```python
from build123d import *

# Parameters (mm, degrees)
SKETCH2_W     = 10
SKETCH2_H     = 5
CHAMFER1_SIZE = 1


with BuildPart() as part:
    # Sketch1 → Revolve1 (revolve)
    with BuildSketch(Plane.XY):
        Polygon((0, 0), (0, 22.5), (110, 22.5), (118.5, 14), (250, 14), (250, 0), align=None)
    revolve(axis=Axis((0, 0, 0), (1, 0, 0)))

    # Sketch2 → Cut-Revolve1 (revolve, cut)
    with BuildSketch(Plane.XY):
        with Locations((235, 11.5)):
            Rectangle(SKETCH2_W, SKETCH2_H)
    revolve(axis=Axis((0, 0, 0), (1, 0, 0)), mode=Mode.SUBTRACT)

    # Chamfer1
    chamfer1_edges = [part.edges().sort_by_distance(p)[0] for p in [
        (230, -14, 0),
        (240, -14, 0),
        (250, -14, 0),
        (0, -22.5, 0),
    ]]
    chamfer(chamfer1_edges, length=CHAMFER1_SIZE)


solid = part.part
```
Could you check a few things on this model? Use its own coordinates, in mm. A direction names the side the tool comes from. Round coordinates to 2 decimals unless told otherwise and drop trailing zeros. Order: outer loops, then holes, each group sorted by start corner. A loop starts at its lowest first (then second) coordinate and runs counter-clockwise, first axis right, second up. Notation, with made-up numbers: M 54,-27.75 L 75,-27.75 A33 cw 75,6.25 Z; hole C 46.5,16 d9. An arc over 180 degrees is marked long. One line per question, with ' | ' between items. Start each with the question number.
(1) Please list where these lines run through material, in increasing order: line 1 along X through (y, z) = (12, -4.5); line 2 along X through (y, z) = (9, 10); line 3 along Z through (x, y) = (35, -6).
(2) Suppose I cut it at C-C on x = 42. List the corners of the cut face in (y, z) for me, then the cut area to 3 significant figures.
(3) For faces 4 (the face through (174.524, 12.932, -5.362)), 5 (the face through (240, -3, 9)), 6 (the face through (0, 0, 0)), which set-ups out of +Z, -Z, +X, -X, +Y, -Y let a thin tool reach every point of the face, with its end or its side?
(4) Thinking about a two-plate mould opening in X: for faces 1 (the face through (230, -3, 9)), 2 (the face through (250, 0, 0)), 3 (the face through (56.263, 10.382, -19.961)), which applies, +X half, -X half, draft (parallel to the pull), parting line (faces both ways), or undercut?
(5) For P1, Ø12, axis at x = 67, z = 6.5, coming from the -Y side; P2, Ø1, axis at x = 111, z = -9, coming from the +Y side; P3, Ø2, axis at x = 194.5, y = -3, coming from the -Z side, each with a flat end and sliding along its axis, tell me the tip position at first contact or that it passes through.
(6) Suppose I cut it at A-A on y = 0. List the corners of the cut face in (x, z) for me, then the cut area to 3 significant figures.
(7) Suppose I cut it at D-D on x = 127. List the corners of the cut face in (y, z) for me.
Geometry results:
1) line 1: 0 to 230, 240 to 250 | line 2: 0 to 229.55, 240.45 to 249.55 | line 3: -21.69 to 21.69
2) outline: C 0,0 d45 | area: 1,590 mm²
3) face 4: +X | face 5: none | face 6: +Z, -Z, -X, +Y, -Y
4) face 1: undercut | face 2: +X half | face 3: draft
5) P1: y = -22.49 | P2: y = 20.12 | P3: z = -13.86
6) outline: M 0,-21.5 L 1,-22.5 L 110,-22.5 L 118.5,-14 L 229,-14 L 230,-13 L 230,-9 L 240,-9 L 240,-13 L 241,-14 L 249,-14 L 250,-13 L 250,13 L 249,14 L 241,14 L 240,13 L 240,9 L 230,9 L 230,13 L 229,14 L 118.5,14 L 110,22.5 L 1,22.5 L 0,21.5 Z | area: 8,840 mm²
7) outline: C 0,0 d28
